Can you work these out from the model? Positions are in its coordinate system, mm. Face numbers are marked on the shaded views. A direction names the side the tool comes from. Coordinates: 2 decimals unless noted, no trailing zeros. Write each loop counter-clockwise with the first axis right and the second up, starting at its lowest first coordinate (ties: lowest second). Pieces come first, ordered by that corner, then holes.
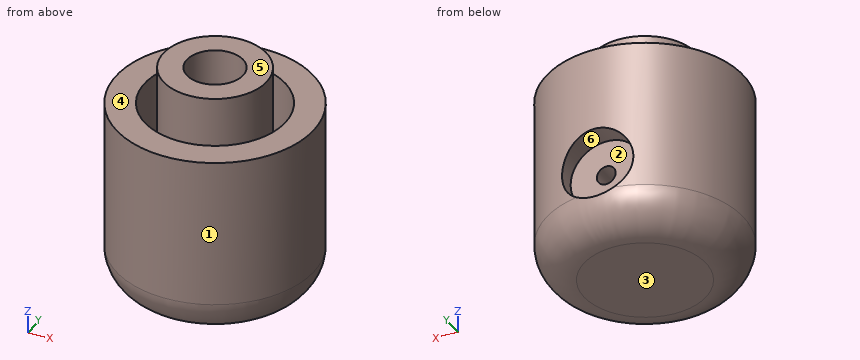
```python
from build123d import *

# Parameters (mm, degrees)
F0_R      = 10.5
F0_R_2    = 7.5
F1_DEPTH  = 20
F2_DEPTH  = 4
F3_R      = 4
F4_R      = 5.5
F4_R_2    = 3
F5_DEPTH  = 20
F6_DEPTH  = 5
F7_R      = 1
F8_DEPTH  = 25
F10_R     = 3.8
F11_DEPTH = 2.5


with BuildPart() as f1:
    # F0 (on Top) → F1 (new body)
    with BuildSketch(Plane.XY):
        Circle(F0_R)
        Circle(F0_R_2, mode=Mode.SUBTRACT)
    extrude(amount=F1_DEPTH)

    # F0 (on Top) → F2 (join)
    with BuildSketch(Plane.XY):
        Circle(F0_R_2)
    extrude(amount=F2_DEPTH)

    # F3
    f3_edges = [f1.edges().sort_by_distance(p)[0] for p in [
        (-10.5, 0, 0),
    ]]
    fillet(f3_edges, radius=F3_R)

    # F4 (on face) → F5 (join)
    with BuildSketch(Plane.XY.offset(4)):
        Circle(F4_R)
        Circle(F4_R_2, mode=Mode.SUBTRACT)
    extrude(amount=F5_DEPTH)

    # F6 (add): a face of the model
    f6_faces = [f1.faces().sort_by_distance(p)[0] for p in [
        (-7.2878679656, 0, 4),
    ]]
    extrude(f6_faces, amount=F6_DEPTH)

    # F7 (on Front) → F8 (cut)
    with BuildSketch(Plane.XZ):
        with Locations((0, 7.2128833695)):
            Circle(F7_R)
    extrude(amount=-F8_DEPTH, mode=Mode.SUBTRACT)

    # F10 (on offset) → F11 (cut)
    with BuildSketch(Plane.XZ.offset(-10.52)):
        with Locations((0, 7.2339284234)):
            Circle(F10_R)
    extrude(amount=F11_DEPTH, mode=Mode.SUBTRACT)


solid = f1.part
```
1. If we section it at A-A, the plane x = 0: List the corners of the cut face in (y, z) for me.
2. If we section it at C-C, the plane y = 0: List the corners of the cut face in (x, z) for me, plus the area to 3 significant figures.
3. Which directions (+Z, -Z, +X, -X, +Y, -Y) give clear straight access to the entire face, cutting with the end or side of a thin tool? Please do the marked faces 4, 5 and 6.
4. If we section it at B-B, the plane z = 12.5: List the corners of the cut face in (x, y) for me, plus the area to 3 significant figures.
5. I'm going to push flat-ended pins straight in: P1, Ø4, axis at x = 2, z = 8, coming from the +Y side; P2, Ø2, axis at x = 8.5, y = -0.5, coming from the +Z side; P3, Ø6, axis at y = -3.5, z = 9, coming from the +X side; P4, Ø5, axis at x = -0.5, y = -1, coming from the +Z side. Where does each tip first touch, or does it pass through?
6. If we section it at D-D, the plane z = 22: List the corners of the cut face in (x, y) for me, plus the area to 3 significant figures.
7. If I drill on L1, parallel to Y at x = 0, z = 17.25; L2, parallel to Y at x = 0, z = 10.5; L3, parallel to X at y = -2.5, z = 17.5, over which ranges is the centre line in solid material (lowest first)?
8. We'd pull the mould along X, two halves only. Please class the marked faces 1, 2 and 3: released by +X, released by -X, zero draft, split by the parting line, or undercut.
Answers:
1. outline: (-10.5, 4) arc R4 ccw to (-6.5, 0) - (6.5, 0) arc R4 ccw to (10.46, 3.43) - (8.02, 3.43) - (8.02, 6.21) - (3, 6.21) - (3, 4) - (-3, 4) - (-3, 24) - (-5.5, 24) - (-5.5, 9) - (-7.5, 9) - (-7.5, 20) - (-10.5, 20) - close; (3, 8.21) - (8.02, 8.21) - (8.02, 11.03) - (10.5, 11.03) - (10.5, 20) - (7.5, 20) - (7.5, 9) - (5.5, 9) - (5.5, 24) - (3, 24) - close
2. outline: (-10.5, 4) arc R4 ccw to (-6.5, 0) - (6.5, 0) arc R4 ccw to (10.5, 4) - (10.5, 20) - (7.5, 20) - (7.5, 9) - (5.5, 9) - (5.5, 24) - (3, 24) - (3, 4) - (-3, 4) - (-3, 24) - (-5.5, 24) - (-5.5, 9) - (-7.5, 9) - (-7.5, 20) - (-10.5, 20) - close
2. area: 293 mm2
3. face 4: +Z
3. face 5: +Z, +X, -X, +Y, -Y
3. face 6: +Y
4. outline: circle Ø21 at (0, 0); circle Ø11 at (0, 0); hole circle Ø15 at (0, 0); hole circle Ø6 at (0, 0)
4. area: 236 mm2
5. P1: stops at y = 10.13
5. P2: stops at z = 20
5. P3: stops at x = 10.49
5. P4: stops at z = 24
6. outline: circle Ø11 at (0, 0); hole circle Ø6 at (0, 0)
6. area: 66.8 mm2
7. L1: y = -10.5 to -7.5, -5.5 to -3, 3 to 5.5, 7.5 to 10.5
7. L2: y = -10.5 to -7.5, -5.5 to -3, 3 to 5.5, 7.5 to 8.02
7. L3: x = -10.2 to -7.07, -4.9 to -1.66, 1.66 to 4.9, 7.07 to 10.2
8. face 1: split by the parting line
8. face 2: undercut
8. face 3: zero draft
